Autodesk Fusion 360 part; units mm, degrees
sketch "Boceto1" plane through (0, 0, 0) normal (0, 0, 1) x (1, 0, 0)
  line L0 (3.25, 0) -> (64.25, 0)
  line L1 (64.25, 6.5) -> (3.25, 6.5)
  circle A0 centre (9.5, 3.25) radius 1.25
  circle A1 centre (3.25, 3.25) radius 3.25
  circle A2 centre (64.25, 3.25) radius 3.25
  circle A3 centre (58, 3.25) radius 1.25
  dimension "d12" = 2.5
  dimension "d14" = 6.5
extrude "Extruir1" add sketch "Boceto1" along normal blind 3 contours L0 L1 A1 A2
extrude "Extruir2" add sketch "Boceto1" along normal blind 10.5 contours A1
extrude "Extruir3" add sketch "Boceto1" along normal blind 10.5 contours A2
extrude "Extruir4" add 1 faces at (3.7107, 2.452, 10.5) along direction (0, 0, 1) blind 1
extrude "Extruir5" add 1 faces at (63.0857, 4.3303, 10.5) along direction (0, 0, 1) blind 1
Work out the finished part from the listing and answer in its coordinate system (mm). A direction names the side the tool comes from. Round coordinates to 2 decimals unless told otherwise and drop trailing zeros. Loops run counter-clockwise (first coordinate to the right, second up) from the corner with the lowest first, then second, coordinate; pieces in that order, holes last. Notation, with made-up numbers: M 21.25,-36.75 L 45.25,-36.75 A28 cw 45.25,-12.75 Z; hole C 20,69.5 d2. An arc over 180 degrees is marked long. One line per question, with ' | ' between items.
Q1. Consider line 1 along Y through (x, z) = (9.5, 2.05); line 2 along Z through (x, y) = (47, 3.25); line 3 along X through (y, z) = (1, 9). Determine where each line is inside the solid, lowest interval first. Write a range as from..to.
Conclusion:
line 1: y = 0..2, 4.5..6.5 | line 2: z = 0..3 | line 3: x = 0.9..5.6, 61.9..66.6
Q2. A tool of negligible diameter and unlimited length cuts with its end or side. For faces 1 (the flat face through (34, 6.5, 1)), 2 (the cylindrical face through (67.35, 2.27, 5.67)), from which of +Z, -Z, +X, -X, +Y, -Y can it reach the whole face along a straight path? Write none if from no direction.
Conclusion:
face 1: +Z, -Z, +X, -X, +Y | face 2: +Z
Q3. Find section D-D, the plane y = 5.75. Give the vertices of the cut face in (x, z), then the cut area to 3 significant figures.
Conclusion:
outline: M 1.17,0 L 66.33,0 L 66.33,11.5 L 62.17,11.5 L 62.17,3 L 5.33,3 L 5.33,11.5 L 1.17,11.5 Z | area: 266 mm2
Q4. The mould has two halves that part along X. Classify faces 3 (the flat face through (33, 3, 0)), 4 (the flat face through (33, 3, 3)): +X half, -X half, draft (parallel to the pull), parting line (faces both ways), or undercut.
Conclusion:
face 3: draft | face 4: undercut
Q5. Find section A-A, the plane x = 9.5. Give the vertices of the cut face in (y, z).
Conclusion:
outline: M 0,0 L 2,0 L 2,3 L 0,3 Z; M 4.5,0 L 6.5,0 L 6.5,3 L 4.5,3 Z
Q6. Find section C-C, the plane z = 6. Give the vertices of the cut face in (x, y).
Conclusion:
outline: C 3.25,3.25 d6.5; C 64.25,3.25 d6.5
Q7. Each of these flat-tipped pins is pushed along its axis until it touches: pin 1 Ø2 at (x, y) = (51.5, 3) entering from +Z; pin 2 Ø1 at (x, y) = (46.5, 5.5) entering from -Z. Where does it stop, or does it pass through?
Conclusion:
pin 1: stops at z = 3 | pin 2: stops at z = 0
Q8. Find section B-B, the plane y = 3.25. Give the vertices of the cut face in (x, z), then the cut area to 3 significant figures.
Conclusion:
outline: M 0,0 L 8.25,0 L 8.25,3 L 6.5,3 L 6.5,11.5 L 0,11.5 Z; M 10.75,0 L 56.75,0 L 56.75,3 L 10.75,3 Z; M 59.25,0 L 67.5,0 L 67.5,11.5 L 61,11.5 L 61,3 L 59.25,3 Z | area: 298 mm2
